```python
from build123d import *

# Parameters (mm, degrees)
F0_R     = 15.875
F1_DEPTH = 31.75
F0_W     = 31.75
F0_H     = 31.75
F2_DEPTH = 92.075
F0_H_2   = 88.9
F3_DEPTH = 73.025


with BuildPart() as f1:
    # F0 (on Top) → F1 (new body)
    with BuildSketch(Plane.XY):
        Polygon((-69.928209, 63.52225), (-127, 63.52225), (-127, 12.72225), (-85.725, 12.72225), (-85.725, -38.07775), (-127, -38.07775), (-127, -88.87775), (-69.928209, -88.87775), (-69.928209, -57.12775), (-69.928209, 31.77225), align=None)
        Polygon((38.021791, 63.52225), (-38.178209, 63.52225), (-38.178209, 31.77225), (-38.178209, -57.12775), (-38.178209, -88.87775), (38.021791, -88.87775), (38.021791, -57.12775), (38.021791, 31.77225), align=None)
        with Locations((0, -12.67775)):
            Circle(F0_R, mode=Mode.SUBTRACT)
        Polygon((127, 63.52225), (69.771791, 63.52225), (69.771791, 31.77225), (69.771791, -57.12775), (69.771791, -88.87775), (127, -88.87775), (127, -40.683407), (85.725, -40.683407), (85.725, 10.116593), (127, 10.116593), align=None)
    extrude(amount=F1_DEPTH)

    # F0 (on Top) → F2 (join)
    with BuildSketch(Plane.XY):
        with Locations((-54.053209, 47.64725)):
            Rectangle(F0_W, F0_H)
        with Locations((-54.053209, -73.00275)):
            Rectangle(F0_W, F0_H)
        with Locations((53.896791, 47.64725)):
            Rectangle(F0_W, F0_H)
        with Locations((53.896791, -73.00275)):
            Rectangle(F0_W, F0_H)
    extrude(amount=F2_DEPTH)

    # F0 (on Top) → F3 (join)
    with BuildSketch(Plane.XY):
        with Locations((-54.053209, -12.67775)):
            Rectangle(F0_W, F0_H_2)
        with Locations((53.896791, -12.67775)):
            Rectangle(F0_W, F0_H_2)
    extrude(amount=F3_DEPTH)


solid = f1.part
```
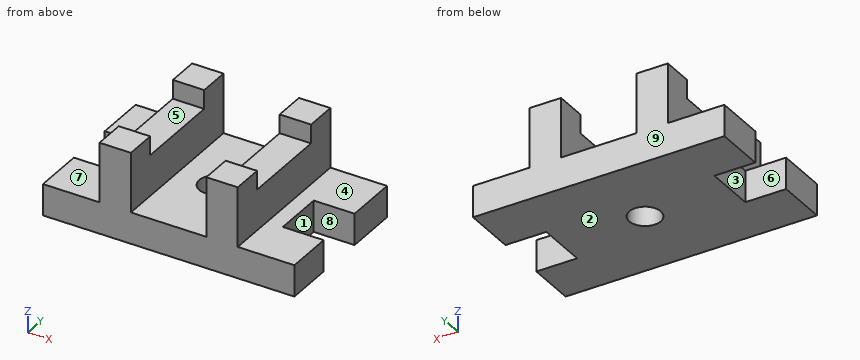
The model under review builds one solid part; all positions refer to its coordinate system, in mm. Face numbers are marked on the shaded views. A direction names the side the tool comes from. Round coordinates to 2 decimals unless told otherwise and drop trailing zeros. Loops run counter-clockwise (first coordinate to the right, second up) from the corner with the lowest first, then second, coordinate; pieces in that order, holes last. Notation, with made-up numbers: (-20, 63) - (1, 63) arc R21 ccw to (1, 82) - close; hole circle Ø4 at (68, 26). An arc over 180 degrees is marked (long way). Use a Markdown table: item, result. Add a question column.
Q1. For probe 1 along Y at (x, z) = (0, 10); probe 2 along X at (y, z) = (7, 52); probe 3 along Y at (x, z) = (-110, 27.5), list the stretches that pass through material, from the lowest coordinate up.
Q2. Machinability: for the marked faces 1, 2, 3, 4 and 5, which of the approach directions +Z, -Z, +X, -X, +Y, -Y give a long, thin tool a straight path to every point of the face, cutting with its end or side? Answer none if there is none.
Q3. Add section D-D (y = 47). State the section outline as (x, z) points (3 decimals), plus the area to 3 significant figures.
Q4. Add section B-B (x = 0). State the section outline as (y, z) points, plus the area to 3 significant figures.
Q5. Insertion check: pin 1 Ø10 at (y, z) = (22.5, 55.5) entering from -X; pin 2 Ø6 at (y, z) = (-53, 52.5) entering from +X; pin 3 Ø3 at (x, y) = (-36.5, -67) entering from +Z; pin 4 Ø12 at (x, y) = (87, -7) entering from -Z. Each pin has a flat end and moves straight along its axis. Give the tip position at first contact, or say it passes through.
Q6. The part is to be moulded in two halves that separate along Y. For the marked faces 6, 7, 8 and 9, say which applies: pulls with the +Y half, pulls with the -Y half, needs draft (parallel to the pull), parting line crosses it, or undercut.
Q7. Add section C-C (z = 77.5). State the section outline as (x, y) points.
Q8. Add section A-A (z = 48). State the section outline as (x, y) points, plus the area to 3 significant figures.
Worked answers:
| question | item | result |
|---|---|---|
| 1 | probe 1 | -88.88 to -28.55, 3.2 to 63.52 |
| 1 | probe 2 | -69.93 to -38.18, 38.02 to 69.77 |
| 1 | probe 3 | -88.88 to -38.08, 12.72 to 63.52 |
| 2 | face 1 | +Z, -Z, +X |
| 2 | face 2 | -Z, +X, -X, +Y, -Y |
| 2 | face 3 | +Z, -Z, -X |
| 2 | face 4 | +Z, +X, +Y, -Y |
| 2 | face 5 | +Z, +X, -X |
| 3 | outline | (-127, 0) - (127, 0) - (127, 31.75) - (69.772, 31.75) - (69.772, 92.075) - (38.022, 92.075) - (38.022, 31.75) - (-38.178, 31.75) - (-38.178, 92.075) - (-69.928, 92.075) - (-69.928, 31.75) - (-127, 31.75) - close |
| 3 | area | 11,900 mm² |
| 4 | outline | (-88.88, 0) - (-28.55, 0) - (-28.55, 31.75) - (-88.88, 31.75) - close; (3.2, 0) - (63.52, 0) - (63.52, 31.75) - (3.2, 31.75) - close |
| 4 | area | 3,830 mm² |
| 5 | pin 1 | x = -69.93 |
| 5 | pin 2 | x = 69.77 |
| 5 | pin 3 | z = 31.75 |
| 5 | pin 4 | z = 0 |
| 6 | face 6 | undercut |
| 6 | face 7 | needs draft |
| 6 | face 8 | undercut |
| 6 | face 9 | pulls with the +Y half |
| 7 | outline | (-69.93, -88.88) - (-38.18, -88.88) - (-38.18, -57.13) - (-69.93, -57.13) - close; (-69.93, 31.77) - (-38.18, 31.77) - (-38.18, 63.52) - (-69.93, 63.52) - close; (38.02, -88.88) - (69.77, -88.88) - (69.77, -57.13) - (38.02, -57.13) - close; (38.02, 31.77) - (69.77, 31.77) - (69.77, 63.52) - (38.02, 63.52) - close |
| 8 | outline | (-69.93, -88.88) - (-38.18, -88.88) - (-38.18, 63.52) - (-69.93, 63.52) - close; (38.02, -88.88) - (69.77, -88.88) - (69.77, 63.52) - (38.02, 63.52) - close |
| 8 | area | 9,680 mm² |
